Build history of the part. All positions in model axes, mm. Round coordinates to 2 decimals unless told otherwise and drop trailing zeros. Write each loop counter-clockwise with the first axis right and the second up, starting at its lowest first coordinate (ties: lowest second). Pieces come first, ordered by that corner, then holes.
Item 1: Band-saw the part on B-B, the plane y = 3.5. Write the cut outline in (x, z).
Item 2: Drop a flat-ended pin along its axis: pin 1 Ø10 at (x, y) = (6, 28.5) entering from -Z. Give the stop position or say it passes through.
Item 3: Wall check: probe 1 along X at (y, z) = (17.5, 0.5). Give the ranges that are in metal, low to high.
Item 4: Band-saw the part on A-A, the plane z = 0.3. Write the cut outline in (x, y), then the cut area to 3 significant figures.
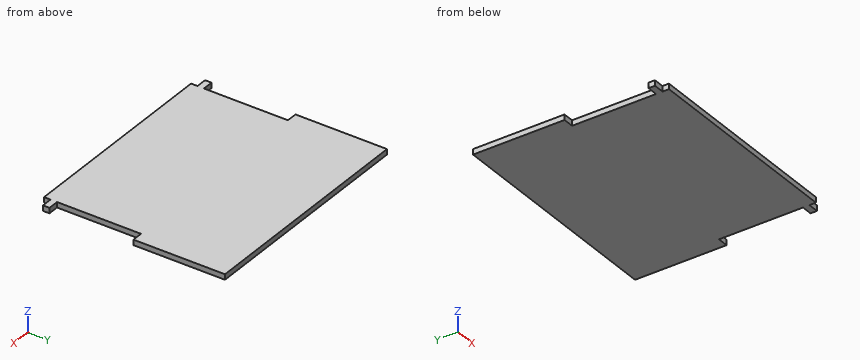
```python
from build123d import *

# Parameters (mm, degrees)
SKETCH037_W     = 21.5
SKETCH037_H     = 35
PAD014_DEPTH    = 1
SKETCH038_W     = 1.2
SKETCH038_H     = 1
SKETCH038_W_2   = 15.6
POCKET024_DEPTH = 2


with BuildPart() as part:
    # Sketch037 → Pad014 (new body)
    with BuildSketch(Plane.XY):
        with Locations((10.75, 17.5)):
            Rectangle(SKETCH037_W, SKETCH037_H)
    extrude(amount=PAD014_DEPTH)

    # Sketch038 (on Face2 of Pad014) → Pocket024 (cut)
    with BuildSketch(Plane.YZ.offset(21.5)):
        with Locations((0.6, 0.5)):
            Rectangle(SKETCH038_W, SKETCH038_H)
        with Locations((10.2, 0.5)):
            Rectangle(SKETCH038_W_2, SKETCH038_H)
    extrude(amount=-POCKET024_DEPTH, mode=Mode.SUBTRACT)

    # Mirrored: part across face of Pocket024


with BuildPart() as part_1:
    add(part.part)
    add(part.part.mirror(Plane(origin=(0, 17.5, 0.5), x_dir=(0, -1, 0), z_dir=(-1, 0, 0))))


solid = part_1.part
```
Results:
1. outline: (-19.5, 0) - (19.5, 0) - (19.5, 1) - (-19.5, 1) - close
2. pin 1: stops at z = 0
3. probe 1: x = -19.5 to 19.5
4. outline: (-21.5, 1.2) - (-19.5, 1.2) - (-19.5, 0) - (19.5, 0) - (19.5, 1.2) - (21.5, 1.2) - (21.5, 2.4) - (19.5, 2.4) - (19.5, 18) - (21.5, 18) - (21.5, 35) - (-21.5, 35) - (-21.5, 18) - (-19.5, 18) - (-19.5, 2.4) - (-21.5, 2.4) - close
4. area: 1,440 mm2
